Could you check a few things on this model? Use its own coordinates, in mm. A direction names the side the tool comes from. Give positions to 0.01 mm unless a question says otherwise; leave off trailing zeros. Order: outer loops, then holes, each group sorted by start corner. A loop starts at its lowest first (then second) coordinate and runs counter-clockwise, first axis right, second up. Notation, with made-up numbers: M 46,26.5 L 54,26.5 A27 ccw 54,52.5 Z; hole C 75,30.5 d1. An arc over 180 degrees is marked long. Use a Markdown table: item, result. Add a question column.
Item 1: If we mould it in two halves opening along Z, with no side actions, what happens to faces 1 (the face through (43, 34, 32.5)), 2 (the face through (0, 25, 15)), 3 (the face through (15, 3.2, 17)), 4 (the face through (43, 34, -2.5))? For each: released by +Z, released by -Z, zero draft, split by the parting line, or undercut.
Item 2: Suppose I cut it at A-A on y = 19. Count the separate pieces of the cut face and the enclosed holes in it, plus the area to 3 significant figures.
Item 3: For faces 5 (the face through (23.63, 60.14, 14.76)), 6 (the face through (42, 16, 26.8)), 7 (the face through (5, 40, 28)), 8 (the face through (10, 12, 28)), 9 (the face through (6.13, 59.86, 14.76)), which set-ups out of +Z, -Z, +X, -X, +Y, -Y let a thin tool reach every point of the face, with its end or its side?
Item 4: I'm going to push flat-ended pins straight in: pin 1 Ø2.5 at (y, z) = (17.5, 28) entering from -X; pin 2 Ø6 at (y, z) = (61, 9.5) entering from -X; pin 3 Ø12 at (y, z) = (22, 10.5) entering from +X. Where does each tip first touch, or does it pass through?
Item 5: Suppose I cut it at D-D on x = 41. Write out the boundary of the cut face in (y, z).
Item 6: Suppose I cut it at C-C on y = 29. Write out the boundary of the cut face in (x, z).
Item 7: If I drill on L1, parallel to X at y = 17.5, z = 17.5; L2, parallel to Z at x = 6, y = 13.5; L3, parallel to X at y = 37, z = 8, over which ranges is the centre line in solid material (lowest first)? Write a range as from..to.
Item 8: Suppose I cut it at B-B on z = 19. Write out the boundary of the cut face in (x, y), plus the area to 3 significant figures.
Autodesk Fusion 360 part; units mm, degrees
sketch "Sketch1" plane through (0, 0, 0) normal (0, 1, 0) x (1, 0, 0)
  line L0 (0, 0) -> (30, 0)
  line L1 (30, 0) -> (30, -30)
  line L2 (30, -30) -> (0, -30)
  line L3 (0, -30) -> (0, 0)
  line L4 (3.2, -3.2) -> (26.8, -3.2)
  line L5 (26.8, -3.2) -> (26.8, -26.8)
  line L6 (26.8, -26.8) -> (3.2, -26.8)
  line L7 (3.2, -26.8) -> (3.2, -3.2)
  line L8 (30, 0) -> (56.8, 0)
  line L9 (56.8, 0) -> (56.8, -30)
  line L10 (56.8, -30) -> (30, -30)
  line L11 (30, -30) -> (30, 0)
  line L12 (30, -3.2) -> (53.6, -3.2)
  line L13 (53.6, -3.2) -> (53.6, -26.8)
  line L14 (53.6, -26.8) -> (30, -26.8)
  dimension "d7" = 30
  dimension "d8" = 30
  dimension "d9" = 3.2
  dimension "d10" = 3.2
  dimension "d11" = 3.2
  dimension "d12" = 3.2
  dimension "d13" = 26.8
  dimension "d14" = 30
  dimension "d15" = 3.2
  dimension "d16" = 3.2
  dimension "d17" = 3.2
extrude "Extrude1" add sketch "Sketch1" along normal blind 50 contours L0 L1 L2 L3 L11 makes body 1
extrude "Extrude2" add sketch "Sketch1" along normal blind 30 contours L1 L8 L9 L10 L11 L12 L13 L14 bodies 1
sketch "Sketch2" plane through (0, 0, 30) normal (0, 0, 1) x (1, 0, 0)
  line L0 (0, 0) -> (56.8, 0)
  line L1 (56.8, 0) -> (56.8, 30)
  line L2 (56.8, 30) -> (30, 30)
  line L3 (30, 30) -> (30, 50)
  line L4 (30, 50) -> (0, 50)
  line L5 (0, 50) -> (0, 0)
  line L6 (10, 21.2) -> (20, 21.2)
  line L7 (20, 21.2) -> (20, 3.2)
  line L8 (20, 3.2) -> (10, 3.2)
  line L9 (10, 3.2) -> (10, 21.2)
  line L10 (5, 44) -> (12.5, 44)
  line L11 (12.5, 44) -> (12.5, 36.5)
  line L12 (12.5, 36.5) -> (5, 36.5)
  line L13 (5, 36.5) -> (5, 44)
  line L14 (17.5, 44) -> (25, 44)
  line L15 (25, 44) -> (25, 36.5)
  line L16 (25, 36.5) -> (17.5, 36.5)
  line L17 (17.5, 36.5) -> (17.5, 44)
  line L18 (31.8, 22) -> (39.3, 22)
  line L19 (39.3, 22) -> (39.3, 14.5)
  line L20 (39.3, 14.5) -> (31.8, 14.5)
  line L21 (31.8, 14.5) -> (31.8, 22)
  line L22 (44.3, 22) -> (51.8, 22)
  line L23 (51.8, 22) -> (51.8, 14.5)
  line L24 (51.8, 14.5) -> (44.3, 14.5)
  line L25 (44.3, 14.5) -> (44.3, 22)
  line L26 (30, 0) -> (0, 0)
  line L27 (0, 50) -> (0, 50.5)
  line L28 (30, 50) -> (32.5, 50)
  line L29 (0, 50) -> (-2.5, 50)
  line L30 (-2.5, 50) -> (15, 70)
  line L31 (15, 70) -> (32.5, 50)
  line L32 (56.8, 30) -> (59.3, 30)
  line L33 (30, 30) -> (27.5, 30)
  line L34 (27.5, 30) -> (41.8, 45)
  line L35 (41.8, 45) -> (59.3, 30)
  dimension "d22" = 7.5
  dimension "d23" = 7.5
  dimension "d24" = 7.5
  dimension "d25" = 7.5
  dimension "d26" = 5
  dimension "d27" = 5
  dimension "d28" = 6
  dimension "d29" = 6
  dimension "d30" = 18
  dimension "d31" = 10
  dimension "d32" = 3.2
  dimension "d33" = 10
  dimension "d34" = 7.5
  dimension "d35" = 7.5
  dimension "d36" = 7.5
  dimension "d37" = 7.5
  dimension "d38" = 5
  dimension "d39" = 5
  dimension "d40" = 8
  dimension "d41" = 8
  dimension "d47" = 0.5
  dimension "d48" = 2.5
  dimension "d49" = 2.5
  dimension "d50" = 20
  dimension "d51" = 17.5
  dimension "d52" = 2.5
  dimension "d53" = 2.5
  dimension "d54" = 15
  dimension "d55" = 17.5
extrude "Extrude3" add sketch "Sketch1" along normal blind 3.2 contours L4 L5 L6 L7 bodies 1
extrude "Extrude4" add sketch "Sketch1" along normal blind 3.2 contours L1 L11 L12 L13 L14 bodies 1
extrude "Extrude5" add sketch "Sketch2" along normal blind 2.5 separate body contours L4 L28 L29 L30 L31 makes body 2
extrude "Extrude6" add sketch "Sketch2" along normal blind 2.5 separate body contours L2 L3 L32 L34 L35 makes body 3
extrude "Extrude7" add sketch "Sketch2" against normal blind 32.5 contours L4 L28 L29 L30 L31 bodies 1 2
extrude "Extrude8" add sketch "Sketch2" against normal blind 32.5 contours L2 L3 L32 L34 L35 bodies 1 3
extrude "Extrude9" add sketch "Sketch2" against normal blind 32.5 contours L3 L33 L34 bodies 1
extrude "Extrude10" add sketch "Sketch2" along normal blind 2.5 contours L3 L33 L34 bodies 1
extrude "Extrude11" cut sketch "Sketch2" against normal blind 3.2 contours L6 L7 L8 L9 bodies 1
extrude "Extrude12" cut sketch "Sketch2" against normal blind 30 contours L10 L11 L12 L13 | L14 L15 L16 L17 | L18 L19 L20 L21 | L22 L23 L24 L25 bodies 1
Findings below:
| question | item | result |
|---|---|---|
| 1 | face 1 | released by +Z |
| 1 | face 2 | zero draft |
| 1 | face 3 | undercut |
| 1 | face 4 | released by -Z |
| 2 | separate pieces | 4 |
| 2 | enclosed holes | 0 |
| 2 | area | 462 mm^2 |
| 3 | face 5 | +Z, -Z, +X, +Y |
| 3 | face 6 | none |
| 3 | face 7 | +Z, -Z |
| 3 | face 8 | +Z |
| 3 | face 9 | +Z, -Z, -X, +Y |
| 4 | pin 1 | stops at x = 0 |
| 4 | pin 2 | stops at x = 4.5 |
| 4 | pin 3 | stops at x = 56.8 |
| 5 | outline | M 0,0 L 30,0 L 30,-2.5 L 44.16,-2.5 L 44.16,32.5 L 30,32.5 L 30,30 L 0,30 Z; hole M 3.2,3.2 L 30,3.2 L 30,26.8 L 3.2,26.8 Z |
| 6 | outline | M 0,0 L 56.8,0 L 56.8,30 L 0,30 Z; hole M 3.2,3.2 L 26.8,3.2 L 26.8,26.8 L 3.2,26.8 Z; hole M 30,3.2 L 53.6,3.2 L 53.6,26.8 L 30,26.8 Z |
| 7 | L1 | x = 0..3.2, 26.8..30, 53.6..56.8 |
| 7 | L2 | z = 0..3.2, 26.8..30 |
| 7 | L3 | x = 0..3.2, 26.8..30, 34.17..51.13 |
| 8 | outline | M -2.5,50 L 0,50 L 0,0 L 56.8,0 L 56.8,30 L 59.3,30 L 41.8,45 L 30,32.62 L 30,50 L 32.5,50 L 15,70 Z; hole M 3.2,3.2 L 26.8,3.2 L 26.8,50 L 3.2,50 Z; hole M 30,3.2 L 53.6,3.2 L 53.6,30 L 30,30 Z |
| 8 | area | 1,150 mm^2 |
